Geometry: see drawing. Coordinates: mm, zero at the bounding-box minimum. Coordinates: 2 decimals unless noted, no trailing zeros. Order: outer loops, then holes, each group sorted by start corner. A loop starts at its lowest first (then second) coordinate and runs counter-clockwise, first axis right, second up. Notation, with made-up numbers: M 58,45.25 L 82,45.25 A12 cw 82,49.25 Z; hole C -19.75,88.5 d10. An arc over 180 degrees is marked long. Answer in a Markdown table with one row per item.
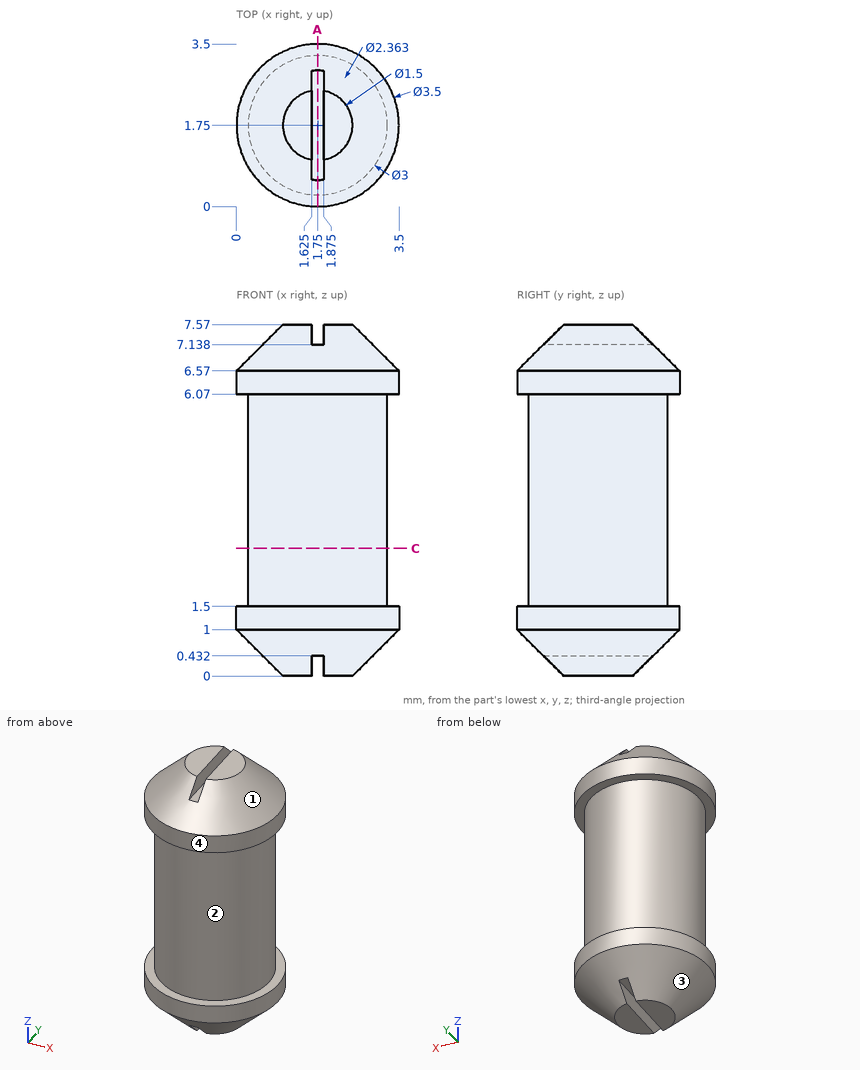
1) Mould query, pull axis Z, two halves, no side actions, for the marked faces 1, 2, 3 and 4. Classes: +Z half, -Z half, draft (parallel to the pull), parting line (faces both ways), or undercut.
Resolved:
| item | result |
|---|---|
| face 1 | +Z half |
| face 2 | undercut |
| face 3 | -Z half |
| face 4 | draft |
2) Cut plane C-C, the plane z = 2.75. Output: boundary loops of the cut face in (x, y).
Resolved:
| item | result |
|---|---|
| outline | C 1.75,1.75 d3 |
3) Cut plane A-A, the plane x = 1.75. Output: boundary loops of the cut face in (y, z).
Resolved:
| item | result |
|---|---|
| outline | M 0,1 L 0.57,0.43 L 2.93,0.43 L 3.5,1 L 3.5,1.5 L 3.25,1.5 L 3.25,6.07 L 3.5,6.07 L 3.5,6.57 L 2.93,7.14 L 0.57,7.14 L 0,6.57 L 0,6.07 L 0.25,6.07 L 0.25,1.5 L 0,1.5 Z |
4) Material intervals for probe 1 along Z at (x, y) = (1, 0.4) (1 decimal); probe 2 along Z at (x, y) = (1, 3.2); probe 3 along Y at (x, z) = (1.2, 2.75) (1 decimal), sorted ascending.
Resolved:
| item | result |
|---|---|
| probe 1 | z = 0.8 to 1.5, 6.1 to 6.8 |
| probe 2 | z = 0.88 to 1.5, 6.07 to 6.69 |
| probe 3 | y = 0.4 to 3.1 |
5) Contact query for flat-ended pins moving along their axis: pin 1 (2 mm diameter, centred on y = 1, z = 6.5, fed in from -X); pin 2 (0.5 mm diameter, centred on y = 1.5, z = 7.5, fed in from -X) (1 decimal); pin 3 (0.5 mm diameter, centred on y = 2, z = 7.5, fed in from +X) (1 decimal); pin 4 (0.5 mm diameter, centred on y = 1.5, z = 0, fed in from +X) (1 decimal). Output: stop coordinate, or through.
Resolved:
| item | result |
|---|---|
| pin 1 | stops at x = 0 |
| pin 2 | stops at x = 0.7 |
| pin 3 | stops at x = 2.8 |
| pin 4 | stops at x = 2.7 |
